```python
from build123d import *

# Parameters (mm, degrees)
SKETCH1_R           = 5.08
SKETCH1_R_2         = 1.4605
BOSS_EXTRUDE1_DEPTH = 3.175
BOSS_EXTRUDE3_START = -3.175
BOSS_EXTRUDE3_DEPTH = 3.175
CUT_EXTRUDE1_DEPTH  = 25.4
FILLET4_R           = 2.54
FILLET5_R           = 12.7
FILLET6_R           = 2.54
FILLET7_R           = 1.27
SKETCH5_R           = 1.4605
CUT_EXTRUDE2_DEPTH  = 25.4


with BuildPart() as part:
    # Sketch1 → Boss-Extrude1 (new body)
    # profile 1 of 3: a face of its own
    with BuildSketch(Plane(origin=(0, 0, 0), x_dir=(1, 0, 0), z_dir=(0, 1, 0))):
        Circle(SKETCH1_R)
        with Locations(Location((0, 0, 0), (0, 0, 270))):
            Circle(SKETCH1_R_2, mode=Mode.SUBTRACT)
    # profile 2 of 3: a face of its own
    with BuildSketch(Plane(origin=(0, 0, 0), x_dir=(1, 0, 0), z_dir=(0, 1, 0))):
        with BuildLine():
            Line((40.720655575, 4.445), (2.459344425, 4.445))
            ThreePointArc((2.459344425, 4.445), (4.376063852, 2.580012628), (5.08, 0))
            ThreePointArc((5.08, 0), (4.376063852, -2.580012628), (2.459344425, -4.445))
            Line((2.459344425, -4.445), (40.720655575, -4.445))
            ThreePointArc((40.720655575, -4.445), (38.1, 0), (40.720655575, 4.445))
        make_face()
    # profile 3 of 3: a face of its own
    with BuildSketch(Plane(origin=(0, 0, 0), x_dir=(1, 0, 0), z_dir=(0, 1, 0))):
        with Locations((43.18, 0)):
            Circle(SKETCH1_R)
        with Locations(Location((43.18, 0, 0), (0, 0, 270))):
            Circle(SKETCH1_R_2, mode=Mode.SUBTRACT)
    extrude(amount=BOSS_EXTRUDE1_DEPTH)

    # Sketch3 → Boss-Extrude3 (add)
    with BuildSketch(Plane(origin=(0, 3.175, 0), x_dir=(1, 0, 0), z_dir=(0, 1, 0)).offset(BOSS_EXTRUDE3_START)):
        with BuildLine():
            Line((35.04998037, 89.507820887), (31.75, 85.645628562))
            ThreePointArc((31.75, 85.645628562), (37.132860765, 53.438748965), (6.35, 42.545))
            Line((6.35, 42.545), (-2.459344425, 4.445))
            ThreePointArc((-2.459344425, 4.445), (0, 5.08), (2.459344425, 4.445))
            Line((2.459344425, 4.445), (35.640655575, 4.445))
            Line((35.640655575, 4.445), (40.720655575, 4.445))
            ThreePointArc((40.720655575, 4.445), (43.226324552, 5.079788779), (45.72, 4.399409051))
            Line((45.72, 4.399409051), (33.02, 41.570560083))
            ThreePointArc((33.02, 41.570560083), (45.702805946, 65.04509807), (35.04998037, 89.507820887))
        make_face()
    extrude(amount=BOSS_EXTRUDE3_DEPTH)

    # Sketch4 → Cut-Extrude1 (cut)
    with BuildSketch(Plane(origin=(0, 3.175, 0), x_dir=(1, 0, 0), z_dir=(0, 1, 0))):
        Polygon((14.401426857, 38.1), (37.998834682, 4.399409051), (27.495360016, 38.1), align=None)
        Polygon((3.175, 0), (35.458834682, 0), (11.089851742, 34.802514411), align=None)
    extrude(amount=-CUT_EXTRUDE1_DEPTH, mode=Mode.SUBTRACT)

    # Fillet4
    fillet4_edges = [part.edges().sort_by_distance(p)[0] for p in [
        (11.089851742, 1.5875, -34.802514411),
        (35.458834682, 1.5875, 0),
        (3.175, 1.5875, 0),
        (14.401426857, 1.5875, -38.1),
        (27.495360016, 1.5875, -38.1),
    ]]
    fillet(fillet4_edges, radius=FILLET4_R)

    # Fillet5
    fillet5_edges = [part.edges().sort_by_distance(p)[0] for p in [
        (33.02, 1.5875, -41.570560083),
    ]]
    fillet(fillet5_edges, radius=FILLET5_R)

    # Fillet6
    fillet6_edges = [part.edges().sort_by_distance(p)[0] for p in [
        (6.35, 1.5875, -42.545),
        (35.04998037, 1.5875, -89.507820887),
        (31.75, 1.5875, -85.645628562),
        (-2.459344425, 1.5875, -4.445),
        (45.72, 1.5875, -4.399409051),
    ]]
    fillet(fillet6_edges, radius=FILLET6_R - 0.0001)  # a hair under: the kernel refuses the full size

    # Fillet7
    fillet7_edges = [part.edges().sort_by_distance(p)[0] for p in [
        (37.998834682, 1.5875, -4.399409051),
    ]]
    fillet(fillet7_edges, radius=FILLET7_R)

    # Sketch5 → Cut-Extrude2 (cut)
    with BuildSketch(Plane(origin=(0, 3.175, 0), x_dir=(1, 0, 0), z_dir=(0, 1, 0))):
        with Locations(Location((11.43, 36.322, 0), (0, 0, 270))):
            Circle(SKETCH5_R)
    extrude(amount=-CUT_EXTRUDE2_DEPTH, mode=Mode.SUBTRACT)


solid = part.part
```
Here's how the part is built. I have some questions about the finished solid (model axes, mm). A direction names the side the tool comes from. Coordinates: 2 decimals unless noted, no trailing zeros. Write each loop counter-clockwise with the first axis right and the second up, starting at its lowest first coordinate (ties: lowest second). Pieces come first, ordered by that corner, then holes. Notation, with made-up numbers: (9, 65) - (65, 65) arc R15 cw to (65, 79) - close; hole circle Ø8 at (1, 53). An arc over 180 degrees is marked (long way). One line per item, written item: value.
1) On a 3-axis mill with a long thin cutter (end or side, diameter ignored), from which of +Z, -Z, +X, -X, +Y, -Y can I reach the whole of each face in a straight line? I mean faces 5 (the flat face through (21, 2, 4.445)), 6 (the flat face through (40.637, 1.565, -19.276)), 7 (the cylindrical face through (17.01, 1.57, -36.7)). Say none if no direction works.
Model answer:
face 5: +Z, +Y, -Y
face 6: +X, +Y, -Y
face 7: +Y, -Y
2) We'd pull the mould along Z, two halves only. Please class faces 1 (the cylindrical face through (47.363, 1.565, 2.883)), 2 (the cylindrical face through (37.439, 1.565, -53.973)), 3 (the flat face through (1.804, 1.565, -22.885)), 4 (the flat face through (21, 0, -25)): pulls with the +Z half, pulls with the -Z half, needs draft (parallel to the pull), parting line crosses it, or undercut.
Model answer:
face 1: parting line crosses it
face 2: undercut
face 3: pulls with the -Z half
face 4: needs draft
3) Suppose I cut it at D-D on z = -54. Write out the boundary of the cut face in (x, y) (3 decimals), and give its area (3 significant figures).
Model answer:
outline: (37.454, 0) - (43.123, 0) - (43.123, 3.175) - (37.454, 3.175) - close
area: 18.0 mm²
4) Suppose I cut it at A-A on x = 43.18. Write out the boundary of the cut face in (y, z) (1 decimal), and give its area (3 significant figures).
Model answer:
outline: (0, -78.5) - (3.2, -78.5) - (3.2, -54.1) - (0, -54.1) - close; (0, -11.8) - (3.2, -11.8) - (3.2, -1.5) - (0, -1.5) - close; (0, 1.5) - (3.2, 1.5) - (3.2, 5.1) - (0, 5.1) - close
area: 122 mm²
5) I need wall thicknesses on line 1 along Z through (x, y) = (27.5, 1.95) (3 decimals); line 2 along X through (y, z) = (2.8, -28); line 3 along X through (y, z) = (1.6, -49). Which ranges of each line are inside material? Lowest first, please.
Model answer:
line 1: z = -44.084 to -37.275, -19.393 to -11.366, 0 to 4.445
line 2: x = 2.99 to 9.54, 15.85 to 21.47, 30.64 to 37.66
line 3: x = 33.82 to 40.32
6) I'm going to push flat-ended pins straight in: P1, Ø1.5, axis at y = 2, z = -14, coming from the -X side; P2, Ø5, axis at x = 41, z = -22.5, coming from the -Y side; P3, Ø1, axis at x = 17.5, y = 1, coming from the +Z side (3 decimals); P4, Ø1, axis at x = 19.5, y = 1, coming from the -Z side. Where does each tip first touch, or does it pass through?
Model answer:
P1: stops at x = -0.42
P2: stops at y = 0
P3: stops at z = 4.445
P4: stops at z = -41.38
7) Suppose I cut it at B-B on x = 0. Write out the boundary of the cut face in (y, z) (1 decimal).
Model answer:
outline: (0, -15.1) - (3.2, -15.1) - (3.2, -1.5) - (0, -1.5) - close; (0, 1.5) - (3.2, 1.5) - (3.2, 5.1) - (0, 5.1) - close
8) Suppose I cut it at C-C on y = 1.75. State how many separate pieces and enclosed holes the cut face has, and give its area (3 significant figures).
Model answer:
separate pieces: 1
enclosed holes: 5
area: 1,370 mm²
